Input: part model. Units: mm. Frame: model coordinates. A direction names the side the tool comes from. Coordinates: 2 decimals unless noted, no trailing zeros. Write each loop counter-clockwise with the first axis right and the second up, starting at its lowest first coordinate (ties: lowest second). Pieces come first, ordered by that corner, then holes. Notation, with made-up numbers: (-10, 33) -> (6, 33) arc R34 ccw to (6, 72) -> close; hole circle Ø8 at (56.5, -20.75). An arc over 180 degrees is marked (long way). One line per question, with ' | ' between items. Start each with the question number.
```python
from build123d import *

# Parameters (mm, degrees)
BOSS_EXTRUDE1_DEPTH = 2


with BuildPart() as part:
    # Sketch1 → Boss-Extrude1 (new body, symmetric)
    with BuildSketch(Plane(origin=(0, 0, 0), x_dir=(1, 0, 0), z_dir=(0, 1, 0))):
        with BuildLine():
            Line((-44, -22), (44, -22))
            ThreePointArc((44, -22), (46.828427125, -20.828427125), (48, -18))
            Line((48, -18), (48, 18))
            ThreePointArc((48, 18), (46.828427125, 20.828427125), (44, 22))
            Line((44, 22), (-44, 22))
            ThreePointArc((-44, 22), (-46.828427125, 20.828427125), (-48, 18))
            Line((-48, 18), (-48, -18))
            ThreePointArc((-48, -18), (-46.828427125, -20.828427125), (-44, -22))
        make_face()
        with BuildLine():
            Line((-38, 10), (-38, -10))
            ThreePointArc((-38, -10), (-40.25, -12.25), (-42.5, -10))
            Line((-42.5, -10), (-42.5, 10))
            ThreePointArc((-42.5, 10), (-40.25, 12.25), (-38, 10))
        make_face(mode=Mode.SUBTRACT)
        with BuildLine():
            Line((42.5, 10), (42.5, -10))
            ThreePointArc((42.5, -10), (40.25, -12.25), (38, -10))
            Line((38, -10), (38, 10))
            ThreePointArc((38, 10), (40.25, 12.25), (42.5, 10))
        make_face(mode=Mode.SUBTRACT)
    extrude(amount=BOSS_EXTRUDE1_DEPTH, both=True)


solid = part.part
```
1) Pull-direction query (Z, two-part tool) for faces 3 (the face through (42.5, 0, 0)), 4 (the face through (-46.859, 0.028, 20.797)), 5 (the face through (48, 0, 0)), 6 (the face through (46.859, 0.028, -20.797)); classes: released by +Z, released by -Z, zero draft, split by the parting line, or undercut.
2) Section C-C, the plane z = -4. Return loops of the section in (x, y).
3) Section A-A, the plane x = -40.25. Return loops of the section in (y, z).
4) Access query for faces 1 (the face through (-48, 0, 0)), 2 (the face through (-40.3, 0.03, -12.25)). Directions: +Z, -Z, +X, -X, +Y, -Y. A direction counts if a zero-diameter tool reaches every point of the face in a straight line with its end or side. Return the directions, or none.
5) Ray query, line 1 (X direction, y = 0.6, z = 4.5); line 2 (Z direction, x = 41, y = 1.85); line 3 (Z direction, x = -38.5, y = -0.1). Return the intervals inside material, ascending.
6) Section B-B, the plane y = -0.1. Return loops of the section in (x, z).
Answer block:
1) face 3: undercut | face 4: released by +Z | face 5: zero draft | face 6: released by -Z
2) outline: (-48, -2) -> (-42.5, -2) -> (-42.5, 2) -> (-48, 2) -> close; (-38, -2) -> (38, -2) -> (38, 2) -> (-38, 2) -> close; (42.5, -2) -> (48, -2) -> (48, 2) -> (42.5, 2) -> close
3) outline: (-2, -22) -> (2, -22) -> (2, -12.25) -> (-2, -12.25) -> close; (-2, 12.25) -> (2, 12.25) -> (2, 22) -> (-2, 22) -> close
4) face 1: +Z, -Z, -X, +Y, -Y | face 2: +Y, -Y
5) line 1: x = -48 to -42.5, -38 to 38, 42.5 to 48 | line 2: z = -22 to -12.12, 12.12 to 22 | line 3: z = -22 to -11.41, 11.41 to 22
6) outline: (-48, -18) arc R4 ccw to (-44, -22) -> (44, -22) arc R4 ccw to (48, -18) -> (48, 18) arc R4 ccw to (44, 22) -> (-44, 22) arc R4 ccw to (-48, 18) -> close; hole (-42.5, -10) arc R2.25 ccw to (-38, -10) -> (-38, 10) arc R2.25 ccw to (-42.5, 10) -> close; hole (38, -10) arc R2.25 ccw to (42.5, -10) -> (42.5, 10) arc R2.25 ccw to (38, 10) -> close
